Build history of the part. All positions in model axes, mm. A direction names the side the tool comes from. Give positions to 0.01 mm unless a question says otherwise; leave off trailing zeros. Loops run counter-clockwise (first coordinate to the right, second up) from the corner with the lowest first, then second, coordinate; pieces in that order, holes last.
1) Wall check: line 1 (X direction, y = 1, z = 0.75); line 2 (Y direction, x = 6, z = -1.25); line 3 (Y direction, x = -17, z = -2). Give the ranges that are in metal, low to high.
2) Two-plate mould, pull along X, no slides. Class faces 1 (the flat face through (-6, -6, -3.175)), 2 (the flat face through (-5.6, -3.2, 0)), 3 (the flat face through (29.843, 23.799, 0.044)): +X half, -X half, draft (parallel to the pull), parting line (faces both ways), or undercut.
3) Band-saw the part on C-C on x = -36. List the corners of the cut face in (y, z) (3 decimals).
4) Band-saw the part on D-D on x = -24. List the corners of the cut face in (y, z) (3 decimals).
5) Band-saw the part on B-B on y = 4. List the corners of the cut face in (x, z) (3 decimals), then the cut area to 3 significant figures.
6) Band-saw the part on A-A on z = 0.5. List the corners of the cut face in (x, y).
7) Flat gauge pins, fed straight in: P1, Ø1.9, axis at x = -1.5, z = 1, coming from the +Y side; P2, Ø2, axis at x = -20, z = 2, coming from the +Y side. Where does each tip first touch, or does it go through?
8) 3-axis set-ups, long thin cutter, end or side, ignore diameter. For faces 4 (the flat face through (-29.843, 23.799, 0.044)), 5 (the flat face through (-6, -6, 3.175)), 6 (the flat face through (16.56, -34.39, 0.04)), 7 (the flat face through (5.6, 3.2, 0)): which of +Z, -Z, +X, -X, +Y, -Y reach the whole face in a straight line?
```python
from build123d import *

# Parameters (mm, degrees)
BOSS_EXTRUDE1_DEPTH = 3.175
CIRPATTERN1_COUNT   = 7
CUT_EXTRUDE1_DEPTH  = 61.984142822


with BuildPart() as part:
    # Sketch1 → Boss-Extrude1 (new, symmetric)
    with BuildSketch(Plane.XY):
        with BuildLine():
            Line((0, 0), (0, 33.1))
            ThreePointArc((0, 33.1), (18.011361269, 36.278515567), (33.696936894, 26.87241046))
            Line((33.696936894, 26.87241046), (0, 0))
        make_face()
    boss_extrude1 = extrude(amount=BOSS_EXTRUDE1_DEPTH, both=True)

    # CirPattern1: Boss-Extrude1 ×7 about axis
    cirpattern1_axis = Axis((0, 0, 0), (0, 0, 1))
    for i in range(1, CIRPATTERN1_COUNT):
        add(boss_extrude1.rotate(cirpattern1_axis, i * 360 / CIRPATTERN1_COUNT))

    # Sketch2 → Cut-Extrude1 (cut, through all)
    with BuildSketch(Plane.XY.offset(3.175)):
        Polygon((7.447818473, 0), (3.723909236, 6.45), (-3.723909236, 6.45), (-7.447818473, 0), (-3.723909236, -6.45), (3.723909236, -6.45), align=None)
    extrude(amount=-CUT_EXTRUDE1_DEPTH, mode=Mode.SUBTRACT)


solid = part.part
```
Findings below:
1. line 1: x = -37.58 to -6.87, 6.87 to 42.24
1. line 2: y = -37.75 to -2.51, 2.51 to 35.68
1. line 3: y = -39.58 to -35.3, -29.91 to 36.82
2. face 1: draft
2. face 2: undercut
2. face 3: +X half
3. outline: (-21.221, -3.175) - (-8.217, -3.175) - (-8.217, 3.175) - (-21.221, 3.175) - close; (-2.315, -3.175) - (23.466, -3.175) - (23.466, 3.175) - (-2.315, 3.175) - close
4. outline: (-28.824, -3.175) - (27.316, -3.175) - (27.316, 3.175) - (-28.824, 3.175) - close
5. outline: (-38.559, -3.175) - (-5.138, -3.175) - (-5.138, 3.175) - (-38.559, 3.175) - close; (5.138, -3.175) - (41.492, -3.175) - (41.492, 3.175) - (5.138, 3.175) - close
5. area: 443 mm2
6. outline: (-42.02, -9.59) arc R26.14 ccw to (-14.36, -29.82) - (-18.7, -38.83) arc R26.14 ccw to (14.36, -29.82) - (18.7, -38.83) arc R26.14 ccw to (32.27, -7.37) - (42.02, -9.59) arc R26.14 ccw to (25.88, 20.64) - (33.7, 26.87) arc R26.14 ccw to (0, 33.1) - (0, 43.1) arc R26.14 ccw to (-25.88, 20.64) - (-33.7, 26.87) arc R26.14 ccw to (-32.27, -7.37) - close; hole (-7.45, 0) - (-3.72, -6.45) - (3.72, -6.45) - (7.45, 0) - (3.72, 6.45) - (-3.72, 6.45) - close
7. P1: stops at y = 43.09
7. P2: stops at y = 34.91
8. face 4: +Z, -Z, +Y
8. face 5: +Z, +X, -X, +Y, -Y
8. face 6: +Z, -Z, -Y
8. face 7: +Z, -Z
